The listing builds one solid part. Answer for the finished solid, in the listing's coordinates (mm). A direction names the side the tool comes from. Coordinates: 2 decimals unless noted, no trailing zeros. Order: outer loops, then holes, each group sorted by start corner. A loop starts at its lowest first (then second) coordinate and runs counter-clockwise, first axis right, second up. Notation, with made-up numbers: (-16.75, -40) -> (-2.75, -40) arc R15 ccw to (-2.75, -24) -> close; hole circle Ø2 at (8.25, -24). An arc over 180 degrees is marked (long way). Answer in a Markdown table with one row per item.
```python
from build123d import *

# Parameters (mm, degrees)
SKETCH1_R                 = 8.89
SKETCH1_R_2               = 6.35
EXTRUDE_THIN1_DEPTH       = 25.4
SKETCH2_R                 = 12.7
SKETCH2_R_2               = 6.35
BOSS_EXTRUDE1_DEPTH       = 2.54
SKETCH3_R                 = 8.89
SKETCH3_R_2               = 6.35
EXTRUDE_THIN2_DEPTH       = 25.4
SKETCH4_R                 = 4.1275
CUT_EXTRUDE1_DEPTH        = 25.4
F_4_CLEARANCE_HOLE1_D     = 3.2639
F_4_CLEARANCE_HOLE1_DEPTH = 25.4
F_4_CLEARANCE_HOLE1_TIP   = 0.980574487
FILLET2_R                 = 1.27
FILLET3_R                 = 1.27


with BuildPart() as part:
    # Sketch1 → Extrude-Thin1 (new body)
    with BuildSketch(Plane(origin=(0, 0, 0), x_dir=(1, 0, 0), z_dir=(0, 1, 0))):
        Circle(SKETCH1_R)
        Circle(SKETCH1_R_2, mode=Mode.SUBTRACT)
    extrude(amount=EXTRUDE_THIN1_DEPTH)

    # Sketch2 → Boss-Extrude1 (add)
    with BuildSketch(Plane(origin=(0, 25.4, 0), x_dir=(1, 0, 0), z_dir=(0, 1, 0))):
        with Locations(Location((0, 0, 0), (0, 0, 270))):
            Circle(SKETCH2_R)
        with Locations(Location((0, 0, 0), (0, 0, 270))):
            Circle(SKETCH2_R_2, mode=Mode.SUBTRACT)
    extrude(amount=BOSS_EXTRUDE1_DEPTH)

    # Sketch3 → Extrude-Thin2 (add)
    with BuildSketch(Plane(origin=(0, 27.94, 0), x_dir=(1, 0, 0), z_dir=(0, 1, 0))):
        Circle(SKETCH3_R)
        Circle(SKETCH3_R_2, mode=Mode.SUBTRACT)
    extrude(amount=EXTRUDE_THIN2_DEPTH)

    # Sketch4 → Cut-Extrude1 (cut)
    with BuildSketch(Plane.XY):
        with Locations(Location((0, 39.37, 0), (0, 0, 90))):
            Circle(SKETCH4_R)
    extrude(amount=-CUT_EXTRUDE1_DEPTH, mode=Mode.SUBTRACT)

    # #4 Clearance Hole1
    with Locations(Plane(origin=(0, 27.94, 0), x_dir=(-1, 0, 0), z_dir=(0, 1, 0))):
        with Locations((-10.795, 0), (0, -10.795), (0, 10.795), (10.795, 0)):
            Hole(F_4_CLEARANCE_HOLE1_D / 2, depth=F_4_CLEARANCE_HOLE1_DEPTH)
            with Locations((0, 0, -(F_4_CLEARANCE_HOLE1_DEPTH + F_4_CLEARANCE_HOLE1_TIP / 2))):  # 118° drill point
                Cone(0, F_4_CLEARANCE_HOLE1_D / 2, F_4_CLEARANCE_HOLE1_TIP, mode=Mode.SUBTRACT)

    # Fillet2
    # the kernel refuses this fillet: 1.27 mm, written as the material it takes off along each edge
    with BuildSketch(Plane(origin=(0, 0, 0), x_dir=(1, 0, 0), z_dir=(0, 0, 1))) as fillet2_piece_1:
        with BuildLine():
            CenterArc((8.89 - FILLET2_R, FILLET2_R), FILLET2_R, 270, 90)
            Line((8.89 - FILLET2_R, 0), (8.89, 0))
            Line((8.89, 0), (8.89, FILLET2_R))
        make_face()
    revolve(axis=Axis((0, 0, 0), (0, 1, 0)), mode=Mode.SUBTRACT)
    with BuildSketch(Plane(origin=(0, 0, 0), x_dir=(1, 0, 0), z_dir=(0, 0, 1))) as fillet2_piece_2:
        with BuildLine():
            CenterArc((6.35 + FILLET2_R, FILLET2_R), FILLET2_R, 180, 90)
            Line((6.35, FILLET2_R), (6.35, 0))
            Line((6.35, 0), (6.35 + FILLET2_R, 0))
        make_face()
    revolve(axis=Axis((0, 0, 0), (0, 1, 0)), mode=Mode.SUBTRACT)

    # Fillet3
    # the kernel refuses this fillet: 1.27 mm, written as the material it takes off along each edge
    with BuildSketch(Plane(origin=(0, 53.34, 0), x_dir=(1, 0, 0), z_dir=(0, 0, 1))) as fillet3_piece_1:
        with BuildLine():
            CenterArc((8.89 - FILLET3_R, -FILLET3_R), FILLET3_R, 0, 90)
            Line((8.89 - FILLET3_R, 0), (8.89, 0))
            Line((8.89, 0), (8.89, -FILLET3_R))
        make_face()
    revolve(axis=Axis((0, 53.34, 0), (0, 1, 0)), mode=Mode.SUBTRACT)
    with BuildSketch(Plane(origin=(0, 53.34, 0), x_dir=(1, 0, 0), z_dir=(0, 0, 1))) as fillet3_piece_2:
        with BuildLine():
            CenterArc((6.35 + FILLET3_R, -FILLET3_R), FILLET3_R, 90, 90)
            Line((6.35 + FILLET3_R, 0), (6.35, 0))
            Line((6.35, 0), (6.35, -FILLET3_R))
        make_face()
    revolve(axis=Axis((0, 53.34, 0), (0, 1, 0)), mode=Mode.SUBTRACT)


solid = part.part
```
(1) A cutting plane is placed at B-B, the plane x = 10. Determine the outline of the cut face in (y, z).
Check values:
| item | result |
|---|---|
| outline | (25.4, -7.83) -> (27.94, -7.83) -> (27.94, -1.43) -> (25.4, -1.43) -> close; (25.4, 1.43) -> (27.94, 1.43) -> (27.94, 7.83) -> (25.4, 7.83) -> close |
(2) Flat-ended cylindrical pins translate along their axes: pin 1 (7.5 mm diameter, centred on x = 2.5, z = -1.5, fed in from -Y); pin 2 (1.5 mm diameter, centred on y = 39.5, z = 2.5, fed in from -X); pin 3 (1.5 mm diameter, centred on y = 29, z = 6.5, fed in from -X); pin 4 (2.5 mm diameter, centred on x = -10.795, z = 0, fed in from +Y). Find the tip coordinate at first contact, or state that the pin passes through.
Check values:
| item | result |
|---|---|
| pin 1 | y = 0.43 |
| pin 2 | x = -8.72 |
| pin 3 | x = -6.78 |
| pin 4 | through |
(3) A cutting plane is placed at D-D, the plane x = -1. Count the separate pieces of the cut face and the enclosed holes in it, then the cut area to 3 significant figures.
Check values:
| item | result |
|---|---|
| separate pieces | 5 |
| enclosed holes | 0 |
| area | 256 mm² |
(4) Find the intervals of material crossed by line 1 along Z through (x, y) = (0, 12); line 2 along X through (y, z) = (12, 5), in increasing order. Write a range as from..to.
Check values:
| item | result |
|---|---|
| line 1 | -8.89..-6.35, 6.35..8.89 |
| line 2 | -7.35..-3.91, 3.91..7.35 |
(5) A cutting plane is placed at C-C, the plane y = 47. Determine the outline of the cut face in (x, z), then the cut area to 3 significant figures.
Check values:
| item | result |
|---|---|
| outline | circle Ø17.78 at (0, 0); hole circle Ø12.7 at (0, 0) |
| area | 122 mm² |
(6) For a pull along Z with two mould halves and no side action, classify faces 1 (the cylindrical face through (-0.35, 26.65, 9.2)), 2 (the flat face through (9, 27.94, -3)), 3 (the cylindrical face through (12.3, 26.65, -0.63)), 4 (the cylindrical face through (-1.93, 13.17, 8.68)) as released by +Z, released by -Z, zero draft, split by the parting line, or undercut.
Check values:
| item | result |
|---|---|
| face 1 | undercut |
| face 2 | zero draft |
| face 3 | undercut |
| face 4 | split by the parting line |
(7) A cutting plane is placed at A-A, the plane z = 10.25. Determine the outline of the cut face in (x, y), then the cut area to 3 significant figures.
Check values:
| item | result |
|---|---|
| outline | (-7.5, 25.4) -> (-1.54, 25.4) -> (-1.54, 27.94) -> (-7.5, 27.94) -> close; (1.54, 25.4) -> (7.5, 25.4) -> (7.5, 27.94) -> (1.54, 27.94) -> close |
| area | 30.3 mm² |
(8) Which of the six approach directions +Z, -Z, +X, -X, +Y, -Y give full straight-line access (tool end or side, diameter ignored) to faces 5 (the cylindrical face through (4.1, 39.84, 7.89)), 6 (the cylindrical face through (-0.181, 35.246, -6.829)), 7 (the flat face through (9, 25.4, -3)), 8 (the cylindrical face through (-0.35, 26.65, -12.39))?
Check values:
| item | result |
|---|---|
| face 5 | +Y |
| face 6 | -Z |
| face 7 | -Y |
| face 8 | +Y, -Y |
